Source: CAD feature listing. Evaluate the final solid. Frame: model axes, mm. A direction names the side the tool comes from. Give positions to 0.01 mm unless a question says otherwise; leave off trailing zeros. Order: outer loops, then holes, each group sorted by start corner. A loop starts at its lowest first (then second) coordinate and runs counter-clockwise, first axis right, second up. Notation, with made-up numbers: (32, 43.25) -> (37, 43.25) arc R23 ccw to (37, 60.25) -> close; hole circle Ø10 at (29, 77). An arc over 180 degrees is marked (long way). Use CSV: the item, a comma, the result in double quotes.
```python
from build123d import *

# Parameters (mm, degrees)
SKETCH1_W           = 77
SKETCH1_H           = 52
SKETCH1_W_2         = 73
SKETCH1_H_2         = 48
BOSS_EXTRUDE1_DEPTH = 4.524
SKETCH2_W           = 77
SKETCH2_H           = 52
BOSS_EXTRUDE2_DEPTH = 2
SKETCH3_R           = 1.75
CUT_EXTRUDE1_DEPTH  = 2
BOSS_EXTRUDE3_START = 3
SKETCH4_R           = 2.75
SKETCH4_R_2         = 1.75
BOSS_EXTRUDE3_DEPTH = 3


with BuildPart() as part:
    # Sketch1 → Boss-Extrude1 (new body)
    with BuildSketch(Plane(origin=(0, 0, 0), x_dir=(1, 0, 0), z_dir=(0, 1, 0))):
        Rectangle(SKETCH1_W, SKETCH1_H)
        Rectangle(SKETCH1_W_2, SKETCH1_H_2, mode=Mode.SUBTRACT)
    extrude(amount=BOSS_EXTRUDE1_DEPTH)

    # Sketch2 → Boss-Extrude2 (add)
    with BuildSketch(Plane.XZ):
        Rectangle(SKETCH2_W, SKETCH2_H)
    extrude(amount=BOSS_EXTRUDE2_DEPTH)

    # Sketch3 → Cut-Extrude1 (cut)
    with BuildSketch(Plane(origin=(0, 0, 0), x_dir=(1, 0, 0), z_dir=(0, 1, 0))):
        with Locations(Location((-33, 20.5, 0), (0, 0, 270))):
            Circle(SKETCH3_R)
        with Locations(Location((33, 20.5, 0), (0, 0, 270))):
            Circle(SKETCH3_R)
        with Locations(Location((33, -20.5, 0), (0, 0, 270))):
            Circle(SKETCH3_R)
        with Locations(Location((-33, -20.5, 0), (0, 0, 270))):
            Circle(SKETCH3_R)
    extrude(amount=-CUT_EXTRUDE1_DEPTH, mode=Mode.SUBTRACT)

    # Sketch4 → Boss-Extrude3 (add)
    # profile 1 of 4: a face of its own
    with BuildSketch(Plane(origin=(0, 0, 0), x_dir=(1, 0, 0), z_dir=(0, 1, 0)).offset(BOSS_EXTRUDE3_START)):
        with Locations(Location((-33, -20.5, 0), (0, 0, 270))):
            Circle(SKETCH4_R)
        with Locations(Location((-33, -20.5, 0), (0, 0, 270))):
            Circle(SKETCH4_R_2, mode=Mode.SUBTRACT)
    # profile 2 of 4: a face of its own
    with BuildSketch(Plane(origin=(0, 0, 0), x_dir=(1, 0, 0), z_dir=(0, 1, 0)).offset(BOSS_EXTRUDE3_START)):
        with Locations(Location((33, -20.5, 0), (0, 0, 270))):
            Circle(SKETCH4_R)
        with Locations(Location((33, -20.5, 0), (0, 0, 270))):
            Circle(SKETCH4_R_2, mode=Mode.SUBTRACT)
    # profile 3 of 4: a face of its own
    with BuildSketch(Plane(origin=(0, 0, 0), x_dir=(1, 0, 0), z_dir=(0, 1, 0)).offset(BOSS_EXTRUDE3_START)):
        with Locations(Location((33, 20.5, 0), (0, 0, 270))):
            Circle(SKETCH4_R)
        with Locations(Location((33, 20.5, 0), (0, 0, 270))):
            Circle(SKETCH4_R_2, mode=Mode.SUBTRACT)
    # profile 4 of 4: a face of its own
    with BuildSketch(Plane(origin=(0, 0, 0), x_dir=(1, 0, 0), z_dir=(0, 1, 0)).offset(BOSS_EXTRUDE3_START)):
        with Locations(Location((-33, 20.5, 0), (0, 0, 270))):
            Circle(SKETCH4_R)
        with Locations(Location((-33, 20.5, 0), (0, 0, 270))):
            Circle(SKETCH4_R_2, mode=Mode.SUBTRACT)
    extrude(amount=-BOSS_EXTRUDE3_DEPTH)


solid = part.part
```
1. Mould query, pull axis X, two halves, no side actions, for faces 1 (the flat face through (38.5, 1, 0)), 2 (the flat face through (-36.5, 2, 0)), 3 (the flat face through (-38.5, 1, 0)). Classes: released by +X, released by -X, zero draft, split by the parting line, or undercut.
Answer below:
face 1,"released by +X"
face 2,"undercut"
face 3,"released by -X"
2. Pin query (flat end, axial travel): P1, Ø4.5, axis at x = -32, z = 21.5, coming from the +Y side; P2, Ø3, axis at x = -33, z = -20.5, coming from the +Y side; P3, Ø24, axis at x = -5, z = -1, coming from the +Y side. Return the tip coordinate at first contact, or that it passes through.
Answer below:
P1,"stops at y = 3"
P2,"passes through"
P3,"stops at y = 0"
3. Section query D-D on z = -8. Return loops of the section in (x, y), plus the area to 3 significant figures.
Answer below:
outline,"(-38.5, -2) -> (38.5, -2) -> (38.5, 4.52) -> (36.5, 4.52) -> (36.5, 0) -> (-36.5, 0) -> (-36.5, 4.52) -> (-38.5, 4.52) -> close"
area,"172 mm²"
4. Access query for faces 4 (the cylindrical face through (34.18, 0.54, 19.21)), 5 (the cylindrical face through (-30.273, 1.521, 20.142)). Directions: +Z, -Z, +X, -X, +Y, -Y. A direction counts if a zero-diameter tool reaches every point of the face in a straight line with its end or side. Return the directions, or none.
Answer below:
face 4,"+Y, -Y"
face 5,"+Y"
5. Section query C-C on x = -33. Return loops of the section in (y, z), plus the area to 3 significant figures.
Answer below:
outline,"(-2, -26) -> (4.52, -26) -> (4.52, -24) -> (0, -24) -> (0, -23.25) -> (3, -23.25) -> (3, -22.25) -> (-2, -22.25) -> close; (-2, -18.75) -> (3, -18.75) -> (3, -17.75) -> (0, -17.75) -> (0, 17.75) -> (3, 17.75) -> (3, 18.75) -> (-2, 18.75) -> close; (-2, 22.25) -> (3, 22.25) -> (3, 23.25) -> (0, 23.25) -> (0, 24) -> (4.52, 24) -> (4.52, 26) -> (-2, 26) -> close"
area,"120 mm²"
6. Section query A-A on y = 1.75. Count the separate pieces of the cut face and the enclosed holes in it, plus the area to 3 significant figures.
Answer below:
separate pieces,"5"
enclosed holes,"5"
area,"557 mm²"
7. Section query B-B on z = -20.5. Return loops of the section in (x, y), plus the area to 3 significant figures.
Answer below:
outline,"(-38.5, -2) -> (-34.75, -2) -> (-34.75, 3) -> (-35.75, 3) -> (-35.75, 0) -> (-36.5, 0) -> (-36.5, 4.52) -> (-38.5, 4.52) -> close; (-31.25, -2) -> (31.25, -2) -> (31.25, 3) -> (30.25, 3) -> (30.25, 0) -> (-30.25, 0) -> (-30.25, 3) -> (-31.25, 3) -> close; (34.75, -2) -> (38.5, -2) -> (38.5, 4.52) -> (36.5, 4.52) -> (36.5, 0) -> (35.75, 0) -> (35.75, 3) -> (34.75, 3) -> close"
area,"170 mm²"
8. Ray query, line 1 along X through (y, z) = (0.5, -2.5); line 2 along X through (y, z) = (0.3, 20.5); line 3 along Z through (x, y) = (13, 0.75). Return the intervals inside material, ascending.
Answer below:
line 1,"x = -38.5 to -36.5, 36.5 to 38.5"
line 2,"x = -38.5 to -36.5, -35.75 to -34.75, -31.25 to -30.25, 30.25 to 31.25, 34.75 to 35.75, 36.5 to 38.5"
line 3,"z = -26 to -24, 24 to 26"
